Part print with two shaded views. Sizes in mm from the minimum x, y, z corner. A direction names the side the tool comes from. Coordinates: 2 decimals unless noted, no trailing zeros. Loops run counter-clockwise (first coordinate to the right, second up) from the corner with the lowest first, then second, coordinate; pieces in that order, holes last.
(1) Flat gauge pins, fed straight in: P1, Ø2.5, axis at y = 7.5, z = 5, coming from the -X side; P2, Ø1, axis at x = 17, y = 11.5, coming from the -Z side; P3, Ø1.5, axis at x = 2.5, z = 5, coming from the -Y side. Where does each tip first touch, or does it go through?
(2) Tool access for the marked faces 4 and 5: list every direction of +Z, -Z, +X, -X, +Y, -Y with a clear straight run to the whole face (end or side of a thin tool).
(3) Slice it at A-A (z = 1.7). Give the cut face in (x, y), and give its area (3 significant figures).
(4) Slice it at C-C (y = 5). Give the cut face in (x, z), and give its area (3 significant figures).
(5) Slice it at B-B (x = 25.4). Give the cut face in (y, z).
(6) Wall check: L1, parallel to Y at x = 5.37, z = 1.2; L2, parallel to Y at x = 10.5, z = 2.4; L3, parallel to X at y = 32, z = 5.3. Give the ranges that are in metal, low to high.
(7) Two-plate mould, pull along X, no slides. Class the marked faces 1, 2 and 3: pulls with the +X half, pulls with the -X half, needs draft (parallel to the pull), parting line crosses it, or undercut.
(8) Slice it at D-D (y = 31.4). Give the cut face in (x, z).
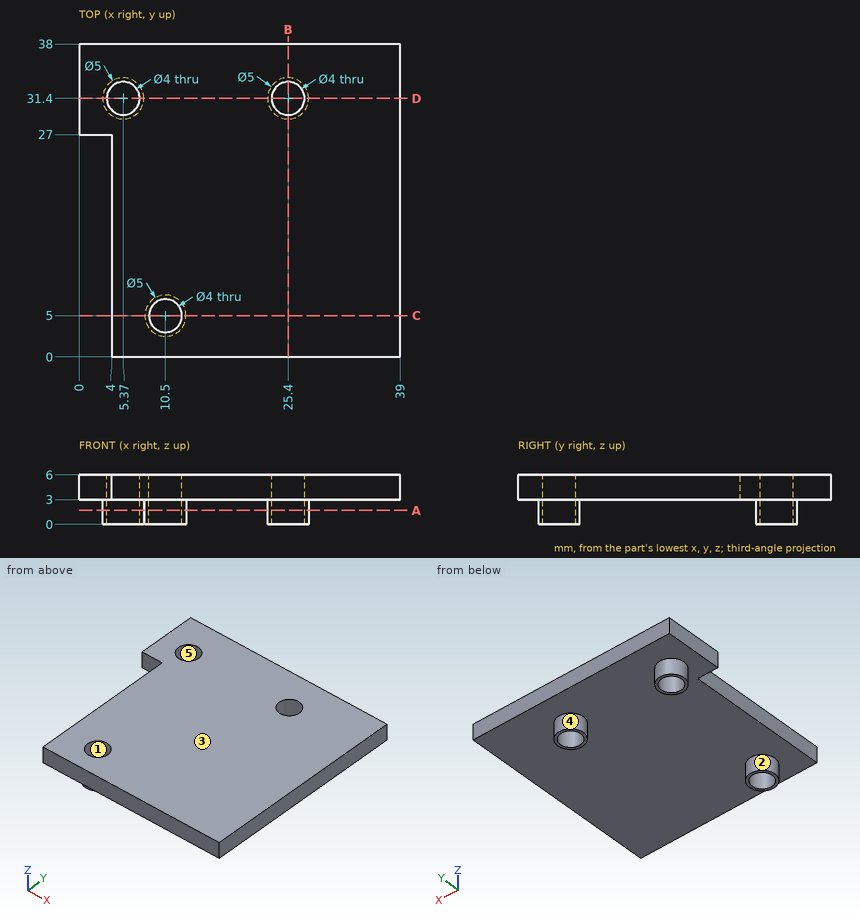
Response values:
1. P1: stops at x = 4
1. P2: stops at z = 3
1. P3: stops at y = 27
2. face 4: -Z
2. face 5: +Z, -Z
3. outline: circle Ø5 at (5.37, 31.4); circle Ø5 at (10.5, 5); circle Ø5 at (25.4, 31.4); hole circle Ø4 at (5.37, 31.4); hole circle Ø4 at (10.5, 5); hole circle Ø4 at (25.4, 31.4)
3. area: 21.2 mm2
4. outline: (4, 3) - (8, 3) - (8, 0) - (8.5, 0) - (8.5, 6) - (4, 6) - close; (12.5, 0) - (13, 0) - (13, 3) - (39, 3) - (39, 6) - (12.5, 6) - close
4. area: 96.0 mm2
5. outline: (0, 3) - (28.9, 3) - (28.9, 0) - (29.4, 0) - (29.4, 6) - (0, 6) - close; (33.4, 0) - (33.9, 0) - (33.9, 3) - (38, 3) - (38, 6) - (33.4, 6) - close
6. L1: y = 28.9 to 29.4, 33.4 to 33.9
6. L2: y = 2.5 to 3, 7 to 7.5
6. L3: x = 0 to 3.46, 7.28 to 23.49, 27.31 to 39
7. face 1: undercut
7. face 2: parting line crosses it
7. face 3: needs draft
8. outline: (0, 3) - (2.87, 3) - (2.87, 0) - (3.37, 0) - (3.37, 6) - (0, 6) - close; (7.37, 0) - (7.87, 0) - (7.87, 3) - (22.9, 3) - (22.9, 0) - (23.4, 0) - (23.4, 6) - (7.37, 6) - close; (27.4, 0) - (27.9, 0) - (27.9, 3) - (39, 3) - (39, 6) - (27.4, 6) - close
